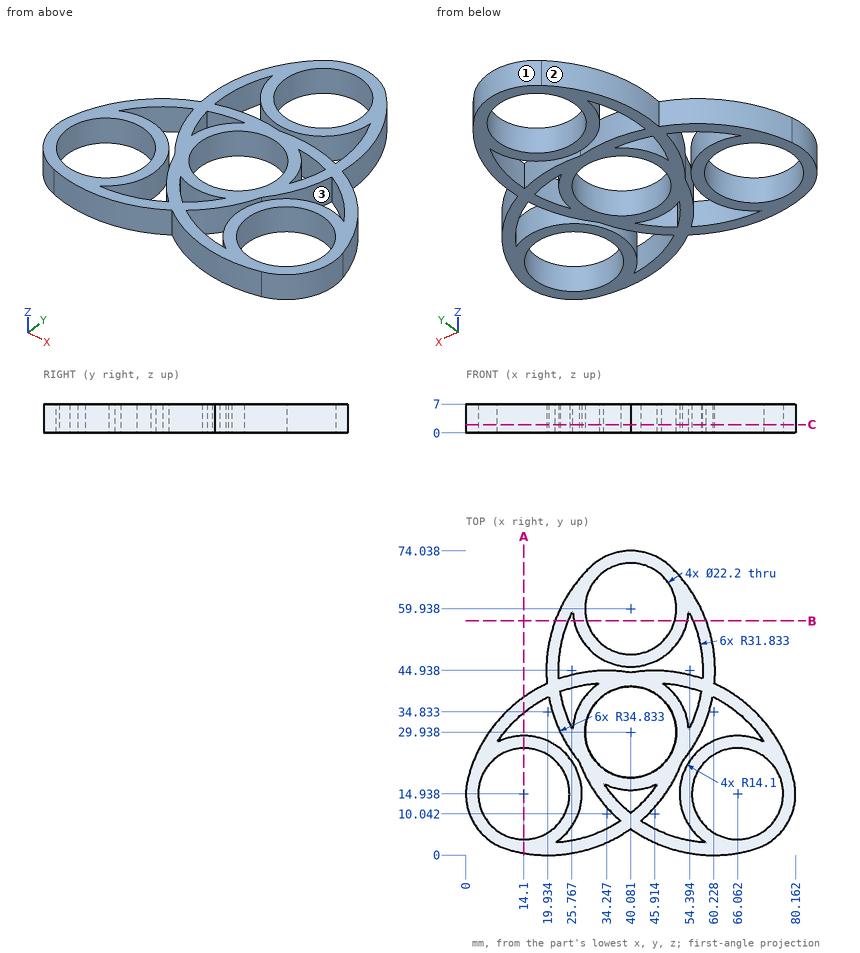
Answer from the drawing. Dimensions are ordinates in mm from the lowest x, y and z of the part. Round coordinates to 2 decimals unless told otherwise and drop trailing zeros. Write each loop counter-clockwise with the first axis right and the second up, starting at its lowest first coordinate (ties: lowest second). Pieces come first, ordered by that corner, then holes. Notation, with made-up numbers: (-39, 37) - (-15, 37) arc R27 ccw to (-15, 68) - close; hole circle Ø9 at (23.25, 44). An arc over 180 degrees is marked (long way). Use a Markdown table: item, result.
(1) Straight lines are drawn through the part: line 1 along Y through (x, z) = (14.1, 2.75); line 2 along Y through (x, z) = (49.5, 5.5) (1 decimal); line 3 along X through (y, z) = (31, 0.5) (1 decimal). For each, find the intervals that lie inside material, in ascending order. Write a range as [from, to].
Reported:
| item | result |
|---|---|
| line 1 | [0.49, 3.84], [26.04, 29.04], [34.69, 38.46] |
| line 2 | [1.7, 4.9], [16.4, 24.1], [35.8, 40.4], [41.7, 44.7], [49.4, 54.1], [65.8, 70.4] |
| line 3 | [6.4, 10.3], [22.5, 25.8], [26, 29], [51.1, 54.1], [54.4, 57.7], [69.9, 73.7] |
(2) The mould has two halves that part along X. Classify the marked faces 1, 2 and 3: released by +X, released by -X, zero draft, split by the parting line, or undercut.
Reported:
| item | result |
|---|---|
| face 1 | split by the parting line |
| face 2 | released by -X |
| face 3 | undercut |
(3) Each of these flat-tipped pins is pushed along its axis until it touches: pin 1 Ø10 at (x, y) = (9.5, 39) entering from -Z; pin 2 Ø1 at (y, z) = (28.5, 2.5) entering from +X; pin 3 Ø1 at (x, z) = (45, 3.5) entering from -Y. Where does it stop, or does it pass through?
Reported:
| item | result |
|---|---|
| pin 1 | z = 0 |
| pin 2 | x = 75.76 |
| pin 3 | y = 3.27 |
(4) The part is cut by section A-A (x = 14.1). Write down the section's boundary in (y, z).
Reported:
| item | result |
|---|---|
| outline | (0.49, 0) - (3.84, 0) - (3.84, 7) - (0.49, 7) - close; (26.04, 0) - (29.04, 0) - (29.04, 7) - (26.04, 7) - close; (34.69, 0) - (38.46, 0) - (38.46, 7) - (34.69, 7) - close |
(5) The part is cut by section B-B (y = 57). Write down the section's boundary in (x, z) (1 decimal).
Reported:
| item | result |
|---|---|
| outline | (21.7, 0) - (24.9, 0) - (24.9, 7) - (21.7, 7) - close; (26.3, 0) - (29.4, 0) - (29.4, 7) - (26.3, 7) - close; (50.8, 0) - (53.9, 0) - (53.9, 7) - (50.8, 7) - close; (55.2, 0) - (58.4, 0) - (58.4, 7) - (55.2, 7) - close |
(6) The part is cut by section C-C (z = 2). State how many separate pieces and enclosed holes the cut face has, then the cut area to 3 significant figures.
Reported:
| item | result |
|---|---|
| separate pieces | 1 |
| enclosed holes | 10 |
| area | 1,620 mm2 |
